The model under review builds one solid part; all positions refer to its coordinate system, in mm. A direction names the side the tool comes from. Coordinates: 2 decimals unless noted, no trailing zeros. Loops run counter-clockwise (first coordinate to the right, second up) from the corner with the lowest first, then second, coordinate; pieces in that order, holes last. Notation, with made-up numbers: M -23,55 L -10,55 A13 cw -10,79 Z; hole C -26,11.5 d3. An arc over 180 degrees is marked long. Return JSON: item names as keys, results as strings.
```python
from build123d import *

# Parameters (mm, degrees)
EXTRUDE_1_DEPTH     = 5
SKETCH_2_R          = 4
CUT_EXTRUDE_1_DEPTH = 6
SKETCH_3_R          = 14
CUT_EXTRUDE_2_DEPTH = 10
CUT_EXTRUDE_4_DEPTH = 224.690634583
FILLET_1_R          = 10
SKETCH_11_R         = 1.6
CUT_EXTRUDE_5_DEPTH = 224.690634583
CUT_EXTRUDE_6_DEPTH = 10


with BuildPart() as part:
    # 草图1 → 凸台-拉伸1 (new body)
    with BuildSketch(Plane(origin=(0, 0, 0), x_dir=(1, 0, 0), z_dir=(0, 1, 0))):
        with BuildLine():
            Line((-0.25, 19.998437439), (199.71875, 22.498242119))
            ThreePointArc((199.71875, 22.498242119), (222.5, 0), (199.71875, -22.498242119))
            Line((199.71875, -22.498242119), (-0.25, -19.998437439))
            ThreePointArc((-0.25, -19.998437439), (-20, 0), (-0.25, 19.998437439))
        make_face()
    extrude(amount=EXTRUDE_1_DEPTH)

    # 草图2 → 切除-拉伸1 (cut)
    with BuildSketch(Plane(origin=(0, 5, 0), x_dir=(1, 0, 0), z_dir=(0, 1, 0))):
        with Locations(Location((0, 0, 0), (0, 0, 270))):
            Circle(SKETCH_2_R)
    extrude(amount=-CUT_EXTRUDE_1_DEPTH, mode=Mode.SUBTRACT)

    # 草图3 → 切除-拉伸2 (cut)
    with BuildSketch(Plane(origin=(0, 5, 0), x_dir=(1, 0, 0), z_dir=(0, 1, 0))):
        with Locations(Location((200, 0, 0), (0, 0, 270))):
            Circle(SKETCH_3_R)
    extrude(amount=-CUT_EXTRUDE_2_DEPTH, mode=Mode.SUBTRACT)

    # 草图10 → 切除-拉伸4 (cut, through all)
    with BuildSketch(Plane(origin=(0, 5, 0), x_dir=(1, 0, 0), z_dir=(0, 1, 0))):
        with BuildLine():
            Line((19.75, 15), (169.71875, 15))
            ThreePointArc((169.71875, 15), (184.427162899, 19.915742901), (199.71875, 22.498242119))
            Line((199.71875, 22.498242119), (-0.25, 19.998437439))
            ThreePointArc((-0.25, 19.998437439), (9.879148371, 18.015973695), (19.75, 15))
        make_face()
        with BuildLine():
            Line((19.75, -15), (169.71875, -15))
            ThreePointArc((169.71875, -15), (184.427162899, -19.915742901), (199.71875, -22.498242119))
            Line((199.71875, -22.498242119), (-0.25, -19.998437439))
            ThreePointArc((-0.25, -19.998437439), (9.879148371, -18.015973695), (19.75, -15))
        make_face()
    extrude(amount=-CUT_EXTRUDE_4_DEPTH, mode=Mode.SUBTRACT)

    # 圆角1
    fillet_1_edges = [part.edges().sort_by_distance(p)[0] for p in [
        (169.71875, 2.5, 15),
        (19.75, 2.5, 15),
        (19.75, 2.5, -15),
        (169.71875, 2.5, -15),
    ]]
    fillet(fillet_1_edges, radius=FILLET_1_R)

    # 草图11 → 切除-拉伸5 (cut, through all)
    with BuildSketch(Plane(origin=(0, 5, 0), x_dir=(1, 0, 0), z_dir=(0, 1, 0))):
        with Locations(Location((160, 0, 0), (0, 0, 270))):
            Circle(SKETCH_11_R)
        with Locations(Location((60, 0, 0), (0, 0, 270))):
            Circle(SKETCH_11_R)
        with Locations(Location((175, 0, 0), (0, 0, 270))):
            Circle(SKETCH_11_R)
        with BuildLine():
            Line((76.800590531, 10), (143.199409469, 10))
            ThreePointArc((143.199409469, 10), (144.693466443, 8.633393255), (143.465138967, 7.023725014))
            Line((143.465138967, 7.023725014), (112.834447973, 1.510200635))
            ThreePointArc((112.834447973, 1.510200635), (110, 1.257133819), (107.165552027, 1.510200635))
            Line((107.165552027, 1.510200635), (76.534861033, 7.023725014))
            ThreePointArc((76.534861033, 7.023725014), (75.306533557, 8.633393255), (76.800590531, 10))
        make_face()
        with BuildLine():
            Line((65, 3.677625158), (65, -3.677625158))
            ThreePointArc((65, -3.677625158), (65.694887325, -5.193105579), (67.296680906, -5.655497864))
            Line((67.296680906, -5.655497864), (98.407090981, -0.988936353))
            ThreePointArc((98.407090981, -0.988936353), (99.258750528, 0), (98.407090981, 0.988936353))
            Line((98.407090981, 0.988936353), (67.296680906, 5.655497864))
            ThreePointArc((67.296680906, 5.655497864), (65.694887325, 5.193105579), (65, 3.677625158))
        make_face()
        with BuildLine():
            Line((155, 3.677625158), (155, -3.677625158))
            ThreePointArc((155, -3.677625158), (154.305112675, -5.193105579), (152.703319094, -5.655497864))
            Line((152.703319094, -5.655497864), (121.592909019, -0.988936353))
            ThreePointArc((121.592909019, -0.988936353), (120.741249472, 0), (121.592909019, 0.988936353))
            Line((121.592909019, 0.988936353), (152.703319094, 5.655497864))
            ThreePointArc((152.703319094, 5.655497864), (154.305112675, 5.193105579), (155, 3.677625158))
        make_face()
        with BuildLine():
            Line((76.534861033, -7.023725014), (107.165552027, -1.510200635))
            ThreePointArc((107.165552027, -1.510200635), (110, -1.257133819), (112.834447973, -1.510200635))
            Line((112.834447973, -1.510200635), (143.465138967, -7.023725014))
            ThreePointArc((143.465138967, -7.023725014), (144.693466443, -8.633393255), (143.199409469, -10))
            Line((143.199409469, -10), (76.800590531, -10))
            ThreePointArc((76.800590531, -10), (75.306533557, -8.633393255), (76.534861033, -7.023725014))
        make_face()
    extrude(amount=-CUT_EXTRUDE_5_DEPTH, mode=Mode.SUBTRACT)

    # 草图12 → 切除-拉伸6 (cut)
    with BuildSketch(Plane(origin=(0, 5, 0), x_dir=(1, 0, 0), z_dir=(0, 1, 0))):
        with BuildLine():
            Line((17.686639759, 9.190462064), (52.313360241, 9.190462064))
            ThreePointArc((52.313360241, 9.190462064), (53.510878101, 8.166743105), (52.685874964, 6.82457346))
            Line((52.685874964, 6.82457346), (39.829631092, 2.67316319))
            ThreePointArc((39.829631092, 2.67316319), (35, 1.91272642), (30.170368908, 2.67316319))
            Line((30.170368908, 2.67316319), (17.314125036, 6.82457346))
            ThreePointArc((17.314125036, 6.82457346), (16.489121899, 8.166743105), (17.686639759, 9.190462064))
        make_face()
        with BuildLine():
            Line((13.279055715, 2.967439032), (13.279055715, -2.967439032))
            ThreePointArc((13.279055715, -2.967439032), (14.040342171, -4.497828215), (15.720146666, -4.813905705))
            Line((15.720146666, -4.813905705), (24.173861919, -2.423097202))
            ThreePointArc((24.173861919, -2.423097202), (26.006717933, 0), (24.173861919, 2.423097202))
            Line((24.173861919, 2.423097202), (15.720146666, 4.813905705))
            ThreePointArc((15.720146666, 4.813905705), (14.040342171, 4.497828215), (13.279055715, 2.967439032))
        make_face()
        with BuildLine():
            Line((56.720944285, 2.967439032), (56.720944285, -2.967439032))
            ThreePointArc((56.720944285, -2.967439032), (55.959657829, -4.497828215), (54.279853334, -4.813905705))
            Line((54.279853334, -4.813905705), (45.826138081, -2.423097202))
            ThreePointArc((45.826138081, -2.423097202), (43.993282067, 0), (45.826138081, 2.423097202))
            Line((45.826138081, 2.423097202), (54.279853334, 4.813905705))
            ThreePointArc((54.279853334, 4.813905705), (55.959657829, 4.497828215), (56.720944285, 2.967439032))
        make_face()
        with BuildLine():
            Line((17.314125036, -6.82457346), (30.170368908, -2.67316319))
            ThreePointArc((30.170368908, -2.67316319), (35, -1.91272642), (39.829631092, -2.67316319))
            Line((39.829631092, -2.67316319), (52.685874964, -6.82457346))
            ThreePointArc((52.685874964, -6.82457346), (53.510878101, -8.166743105), (52.313360241, -9.190462064))
            Line((52.313360241, -9.190462064), (17.686639759, -9.190462064))
            ThreePointArc((17.686639759, -9.190462064), (16.489121899, -8.166743105), (17.314125036, -6.82457346))
        make_face()
    extrude(amount=-CUT_EXTRUDE_6_DEPTH, mode=Mode.SUBTRACT)


solid = part.part
```
1. To check wall thickness, follow line 1 (X direction, y = 2.6, z = 9.5); line 2 (Z direction, x = 52, y = 2.1); line 3 (Z direction, x = 67, y = 1.55). State the ranges of each line that lie inside material, in increasing order.
Check values:
{"line 1": "-17.6 to 75.68, 144.32 to 189.72, 210.28 to 220.4", "line 2": "-15 to -9.19, -6.6 to -4.17, 4.17 to 6.6, 9.19 to 15", "line 3": "-15 to -5.68, 5.68 to 15"}
2. Add section A-A on x = 203. Give the boundary of the cut face in (y, z), plus the area to 3 significant figures.
Check values:
{"outline": "M 0,-22.3 L 5,-22.3 L 5,-13.67 L 0,-13.67 Z; M 0,13.67 L 5,13.67 L 5,22.3 L 0,22.3 Z", "area": "86.2 mm²"}
3. Machinability: for faces 3 (the face through (19.888, 2.535, 3.635)), 4 (the face through (169.61, 2.465, -15.176)), which of the approach directions +Z, -Z, +X, -X, +Y, -Y give a long, thin tool a straight path to every point of the face, cutting with its end or side? Answer none if there is none.
Check values:
{"face 3": "+Y, -Y", "face 4": "-Z, +Y, -Y"}
4. The part is to be moulded in two halves that separate along X. For faces 1 (the face through (103, 5, 0)), 2 (the face through (26.006, 2.535, 0.046)), say which applies: released by +X, released by -X, zero draft, split by the parting line, or undercut.
Check values:
{"face 1": "zero draft", "face 2": "undercut"}
5. Add section B-B on y = 2.4. State how many separate pieces and enclosed holes the cut face has, plus the area to 3 significant figures.
Check values:
{"separate pieces": "1", "enclosed holes": "13", "area": "5,300 mm²"}
6. Insertion check: pin 1 Ø1.5 at (x, y) = (136.5, 2.5) entering from +Z; pin 2 Ø1.5 at (y, z) = (2.5, 1.5) entering from +X; pin 3 Ø2.5 at (x, y) = (116.5, 3.5) entering from -Z. Each pin has a flat end and moves straight along its axis. Give the tip position at first contact, or say it passes through.
Check values:
{"pin 1": "z = 15", "pin 2": "x = 222.49", "pin 3": "z = -15"}
